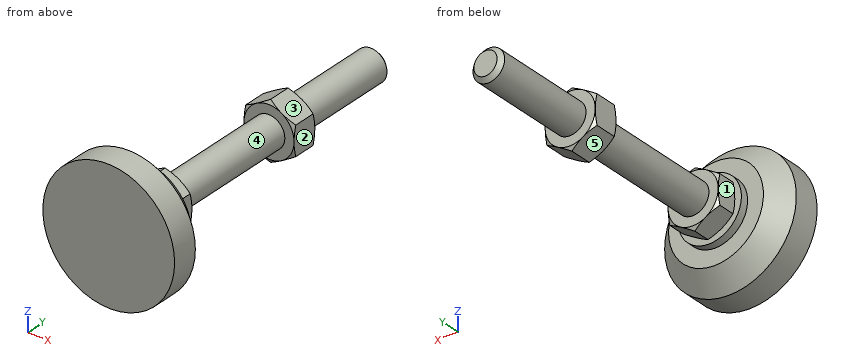
from build123d import *

# Parameters (mm, degrees)
EXTRUDE_1_DEPTH = 8
EXTRUDE_2_DEPTH = 10


with BuildPart() as part:
    # Эскиз1 → Повернуть1 (revolve)
    with BuildSketch(Plane.XY, mode=Mode.PRIVATE) as revolve_1_sk:
        Polygon((0, 0), (-25, 0), (-25, 10), (-18, 17), (-12, 17), (-12, 20), (-6, 20), (-6, 28), (-6, 126.4), (-4.4, 128), (0, 128), align=None)
    revolve(revolve_1_sk.sketch.rotate(Axis((0, 0, 0), (0, 1, 0)), 180), axis=Axis((0, 0, 0), (0, 1, 0)))  # turned: the seam where the file's is

    # Эскиз2 → Бобышка-Вытянуть1 (add)
    with BuildSketch(Plane(origin=(0, 20, 0), x_dir=(1, 0, 0), z_dir=(0, 1, 0))):
        Polygon((0, 10.969655115), (-9.5, 5.484827557), (-9.5, -5.484827557), (0, -10.969655115), (9.5, -5.484827557), (9.5, 5.484827557), align=None)
    extrude(amount=EXTRUDE_1_DEPTH)

    # Эскиз3 → Бобышка-Вытянуть2 (add)
    with BuildSketch(Plane(origin=(0, 77.2, 0), x_dir=(1, 0, 0), z_dir=(0, 1, 0))):
        Polygon((9.5, 5.484827557), (0, 10.969655115), (-9.5, 5.484827557), (-9.5, -5.484827557), (0, -10.969655115), (9.5, -5.484827557), align=None)
    extrude(amount=EXTRUDE_2_DEPTH)

    # Эскиз4 → Вырез-Повернуть2 (revolve, cut)
    with BuildSketch(Plane.XY, mode=Mode.PRIVATE) as cut_revolve_2_sk:
        Polygon((-18.160254038, 87.2), (-9.5, 87.2), (-18.160254038, 82.2), align=None)
        Polygon((-18.160254038, 77.2), (-18.160254038, 82.2), (-9.5, 77.2), align=None)
        Polygon((-16.42820323, 28), (-16.42820323, 24), (-9.5, 28), align=None)
        Polygon((-16.42820323, 24), (-16.42820323, 20), (-9.5, 20), align=None)
    revolve(cut_revolve_2_sk.sketch.rotate(Axis((0, 128, 0), (0, -1, 0)), 180), axis=Axis((0, 128, 0), (0, -1, 0)), mode=Mode.SUBTRACT)  # turned: the seam where the file's is


solid = part.part
Geometry check sheet. Reference: the model listing, model coordinates, mm. Face numbers are marked on the shaded views. A direction names the side the tool comes from. Give positions to 0.01 mm unless a question says otherwise; leave off trailing zeros. Order: outer loops, then holes, each group sorted by start corner. A loop starts at its lowest first (then second) coordinate and runs counter-clockwise, first axis right, second up. Notation, with made-up numbers: (82, -11.5) - (103, -11.5) arc R23 cw to (103, 4.5) - close; hole circle Ø6 at (50.25, 79.25). An arc over 180 degrees is marked (long way). Use one line per item in the form item = value.
1) Sectioned sample at A-A (y = 94). Record the boundary of the cut face in (x, z), and give its area (3 significant figures).
Working result:
outline = circle Ø12 at (0, 0)
area = 113 mm^2
2) Material ranges on probe 1 along Y at (x, z) = (6.5, 15); probe 2 along Z at (x, y) = (0, 50); probe 3 along X at (y, z) = (36, 0.5), recorded low to high. Write a range as from..to.
Working result:
probe_1 = 0..17
probe_2 = -6..6
probe_3 = -5.98..5.98
3) Access from +Z, -Z, +X, -X, +Y, -Y to the whole of each face (thin tool, end or side, straight path). Record for the marked faces 1, 2, 3, 4 and 5.
Working result:
face_1 = +Z, -Z, -X, +Y
face_2 = +Z, -Z, +X, +Y
face_3 = +Z, +X, +Y
face_4 = none
face_5 = -Z, -X, +Y
4) Depth check by flat-ended pin: pin 1 Ø2.5 at (y, z) = (23, -2.5) entering from -X; pin 2 Ø2.5 at (y, z) = (26, 2) entering from +X; pin 3 Ø1 at (x, y) = (5, 27) entering from +Z. Enter the tip coordinate at first touch or a pass-through.
Working result:
pin_1 = -9.5
pin_2 = 9.5
pin_3 = 8.37
